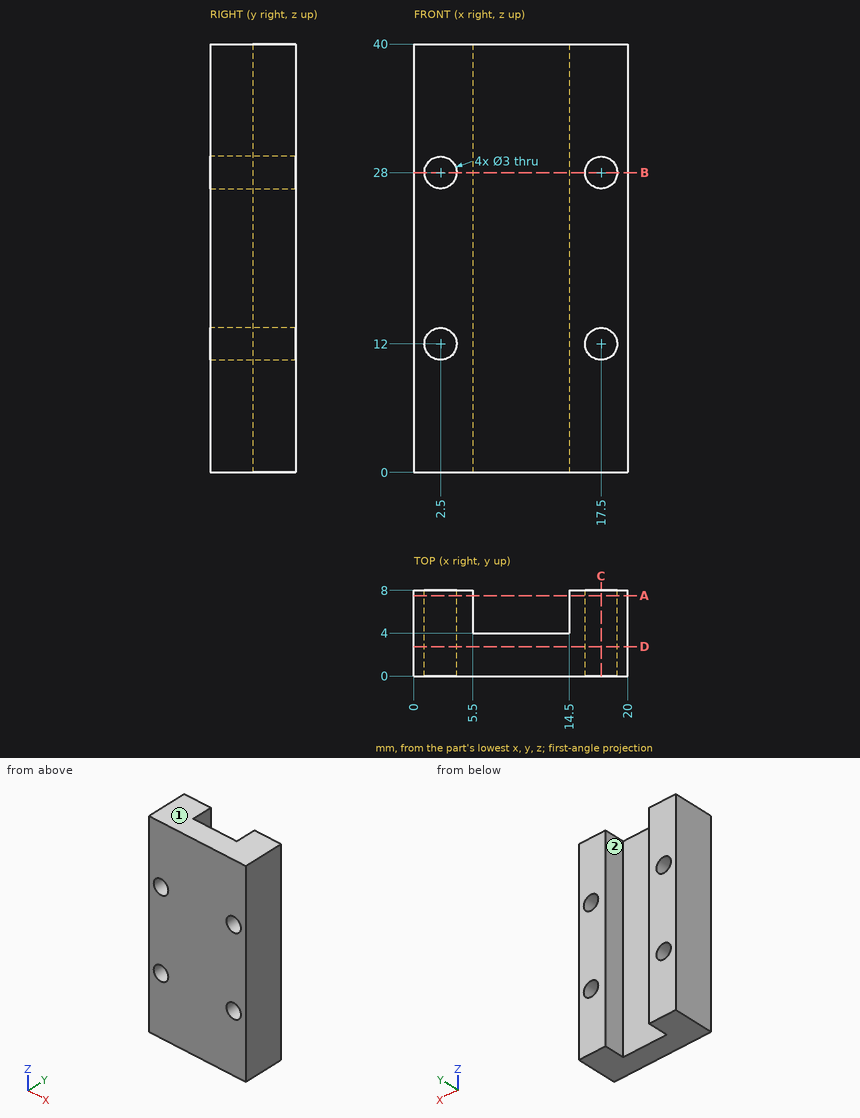
Design review of the part shown in the three views and the two pictorial views. Dimensions are in mm from the part's minimum x, y and z. A direction names the side the tool comes from. Coordinates: 2 decimals unless noted, no trailing zeros. Loops run counter-clockwise (first coordinate to the right, second up) from the corner with the lowest first, then second, coordinate; pieces in that order, holes last.
Q1. We need section B-B on z = 28. State the section outline as (x, y) points, and give its area (3 significant figures).
Reported:
outline: (0, 0) - (1, 0) - (1, 8) - (0, 8) - close; (4, 0) - (16, 0) - (16, 8) - (14.5, 8) - (14.5, 4) - (5.5, 4) - (5.5, 8) - (4, 8) - close; (19, 0) - (20, 0) - (20, 8) - (19, 8) - close
area: 76.0 mm2
Q2. We need section C-C on x = 17.5. State the section outline as (y, z) points.
Reported:
outline: (0, 0) - (8, 0) - (8, 10.5) - (0, 10.5) - close; (0, 13.5) - (8, 13.5) - (8, 26.5) - (0, 26.5) - close; (0, 29.5) - (8, 29.5) - (8, 40) - (0, 40) - close
Q3. We need section D-D on y = 2.75. State the section outline as (x, z) points, and give its area (3 significant figures).
Reported:
outline: (0, 0) - (20, 0) - (20, 40) - (0, 40) - close; hole circle Ø3 at (2.5, 12); hole circle Ø3 at (2.5, 28); hole circle Ø3 at (17.5, 12); hole circle Ø3 at (17.5, 28)
area: 772 mm2
Q4. Tool access review of the marked faces 1 and 2: name each direction out of +Z, -Z, +X, -X, +Y, -Y from which nothing blocks a thin tool from reaching the whole face with its end or side.
Reported:
face 1: +Z, +X, -X, +Y, -Y
face 2: +Z, -Z, +Y
Q5. To check wall thickness, follow line 1 (X direction, y = 3.25, z = 28); line 2 (Z direction, x = 17.75, y = 1.25); line 3 (X direction, y = 6, z = 12). State the ranges of each line that lie inside material, in increasing order.
Reported:
line 1: x = 0 to 1, 4 to 16, 19 to 20
line 2: z = 0 to 10.52, 13.48 to 26.52, 29.48 to 40
line 3: x = 0 to 1, 4 to 5.5, 14.5 to 16, 19 to 20
Q6. For pin 1 (1.5 mm diameter, centred on y = 3.5, z = 13.5, fed in from -X); pin 2 (4.5 mm diameter, centred on x = 11, z = 27.5, fed in from +Y); pin 3 (2.5 mm diameter, centred on x = 17.5, z = 12, fed in from -Y), all flat-tipped, find the tip position at first contact; note any pin that passes through.
Reported:
pin 1: stops at x = 0
pin 2: stops at y = 4
pin 3: passes through
Q7. We need section A-A on y = 7.5. State the section outline as (x, z) points.
Reported:
outline: (0, 0) - (5.5, 0) - (5.5, 40) - (0, 40) - close; (14.5, 0) - (20, 0) - (20, 40) - (14.5, 40) - close; hole circle Ø3 at (2.5, 12); hole circle Ø3 at (2.5, 28); hole circle Ø3 at (17.5, 12); hole circle Ø3 at (17.5, 28)
